For this review, take the finished solid that the model builds, in its own axes (mm). A direction names the side the tool comes from. Coordinates: 2 decimals unless noted, no trailing zeros. Loops run counter-clockwise (first coordinate to the right, second up) from the corner with the lowest first, then second, coordinate; pieces in that order, holes last.
1. Take a section at A-A, the plane z = 0. State the section outline as (x, y) points, then the cut area to 3 significant figures.
2. Take a section at C-C, the plane y = -16. State the section outline as (x, z) points, then the cut area to 3 significant figures.
3. Take a section at B-B, the plane x = -58. State the section outline as (y, z) points, then the cut area to 3 significant figures.
4. Take a section at D-D, the plane z = 20. State the section outline as (x, y) points, then the cut area to 3 significant figures.
5. To check wall thickness, follow probe 1 along X at (y, z) = (9.5, -12); probe 2 along Z at (x, y) = (-45.5, 0); probe 3 along Z at (x, y) = (-42.5, 9). State the ranges of each line that lie inside material, in increasing order.
6. Clearance check with flat-ended pins moving along their axes: P1, Ø1, axis at y = 9.5, z = 17, coming from the -X side; P2, Ø10, axis at x = -150.5, z = 1, coming from the +Y side; P3, Ø3, axis at x = -83.5, z = 9.5, coming from the -Y side. State where each tip first meets the part, or that it passes through.
7. Machinability: for faces 1 (the face through (0, 0, 0)), 2 (the face through (-95.22, 12.47, -5.17)), which of the approach directions +Z, -Z, +X, -X, +Y, -Y give a long, thin tool a straight path to every point of the face, cutting with its end or side? Answer none if there is none.
```python
from build123d import *

# Parameters (mm, degrees)
F0_R     = 13.5
F1_DEPTH = 190
F0_R_2   = 25
F2_DEPTH = 5


with BuildPart() as f1:
    # F0 (on Right) → F1 (new body)
    with BuildSketch(Plane.YZ):
        Circle(F0_R)
    extrude(amount=-F1_DEPTH)

    # F0 (on Right) → F2 (join)
    with BuildSketch(Plane.YZ):
        Circle(F0_R_2)
        Circle(F0_R, mode=Mode.SUBTRACT)
    extrude(amount=-F2_DEPTH)

    # F4 (on face) → F5 (revolve, cut)
    with BuildSketch(Plane(origin=(0, 0, 0), x_dir=(-1, 0, 0), z_dir=(0, 1, 0))):
        Polygon((190, 13.5), (188, 13.5), (190, 10.035898), align=None)
    revolve(axis=Axis((-95, 0, 0), (-1, 0, 0)), mode=Mode.SUBTRACT)


solid = f1.part
```
Results list:
1. outline: (-190, -10.04) - (-188, -13.5) - (-5, -13.5) - (-5, -25) - (0, -25) - (0, 25) - (-5, 25) - (-5, 13.5) - (-188, 13.5) - (-190, 10.04) - close
1. area: 5,240 mm2
2. outline: (-5, -19.21) - (0, -19.21) - (0, 19.21) - (-5, 19.21) - close
2. area: 192 mm2
3. outline: circle Ø27 at (0, 0)
3. area: 573 mm2
4. outline: (-5, -15) - (0, -15) - (0, 15) - (-5, 15) - close
4. area: 150 mm2
5. probe 1: x = -5 to 0
5. probe 2: z = -13.5 to 13.5
5. probe 3: z = -10.06 to 10.06
6. P1: stops at x = -5
6. P2: stops at y = 13.5
6. P3: stops at y = -10.87
7. face 1: +Z, -Z, +X, +Y, -Y
7. face 2: -X
